The figure shows three views and two pictorial views of one solid part (mm, origin at its lowest corner). Answer the questions. A direction names the side the tool comes from. Coordinates: 2 decimals unless noted, no trailing zeros. Order: outer loops, then holes, each group sorted by start corner. A loop starts at its lowest first (then second) coordinate and runs counter-clockwise, first axis right, second up. Notation, with made-up numbers: (50.25, 75.5) - (74.25, 75.5) arc R16 ccw to (74.25, 100.5) - close; hole circle Ø3 at (83.25, 0.25). An arc over 180 degrees is marked (long way). Use one line per item in the form item = value.
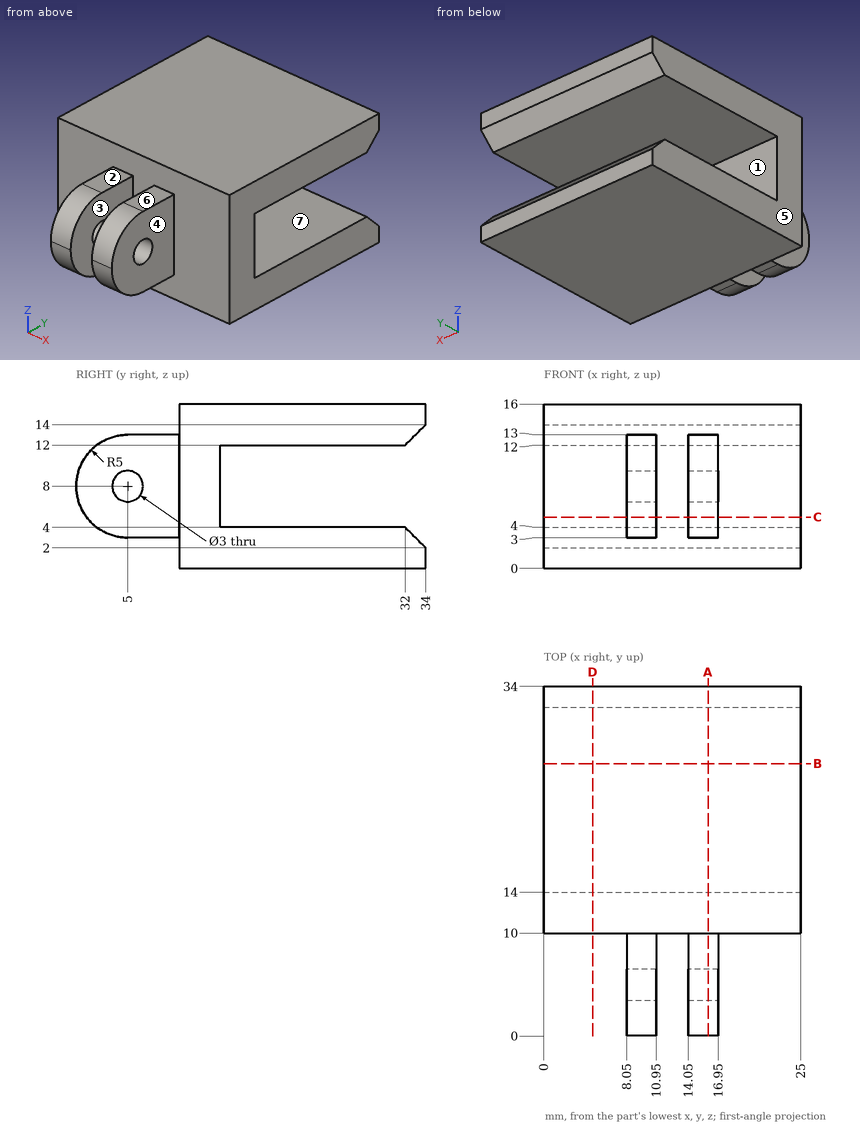
(1) Section B-B, the plane y = 26.5 is taken. Write down the section's boundary in (x, z), then the cut area to 3 significant figures.
Answer list:
outline = (0, 0) - (25, 0) - (25, 4) - (0, 4) - close; (0, 12) - (25, 12) - (25, 16) - (0, 16) - close
area = 200 mm2
(2) Given pin 1 Ø8 at (x, z) = (17, 7) entering from +Y; pin 2 Ø3 at (y, z) = (7.5, 6.5) entering from +X; pin 3 Ø0.9 at (x, y) = (15.5, 8.5) entering from -Z; pin 4 Ø9 at (x, y) = (11.5, 25) entering from -Z, each flat-ended and moving along its own axis, determine where each tip first touches the part or whether it passes through.
Answer list:
pin_1 = 33
pin_2 = 16.95
pin_3 = 3
pin_4 = 0
(3) Section A-A, the plane x = 16 is taken. Write down the section's boundary in (y, z).
Answer list:
outline = (5, 3) - (10, 3) - (10, 0) - (34, 0) - (34, 2) - (32, 4) - (14, 4) - (14, 12) - (32, 12) - (34, 14) - (34, 16) - (10, 16) - (10, 13) - (5, 13) arc R5 ccw to start; hole circle Ø3 at (5, 8)
(4) Which of the six approach directions +Z, -Z, +X, -X, +Y, -Y give full straight-line access (tool end or side, diameter ignored) to the marked faces 1, 2, 3 and 4?
Answer list:
face_1 = +X, -X, +Y
face_2 = +Z, +X, -X, -Y
face_3 = +Z, -Z, -Y
face_4 = +Z, -Z, +X, -Y
(5) The mould has two halves that part along Z. Classify the marked faces 5, 6 and 7: +Z half, -Z half, draft (parallel to the pull), parting line (faces both ways), or undercut.
Answer list:
face_5 = draft
face_6 = +Z half
face_7 = undercut
(6) Section D-D, the plane x = 4.75 is taken. Write down the section's boundary in (y, z), then the cut area to 3 significant figures.
Answer list:
outline = (10, 0) - (34, 0) - (34, 2) - (32, 4) - (14, 4) - (14, 12) - (32, 12) - (34, 14) - (34, 16) - (10, 16) - close
area = 220 mm2
(7) Straight lines are drawn through the part: L1, parallel to Z at x = 13.25, y = 31.5; L2, parallel to X at y = 9, z = 7.5; L3, parallel to Y at x = 23, z = 7.5. For each, find the intervals that lie inside material, in ascending order.
Answer list:
L1 = 0 to 4, 12 to 16
L2 = 8.05 to 10.95, 14.05 to 16.95
L3 = 10 to 14
(8) Section C-C, the plane z = 5 is taken. Write down the section's boundary in (x, y).
Answer list:
outline = (0, 10) - (8.05, 10) - (8.05, 1) - (10.95, 1) - (10.95, 10) - (14.05, 10) - (14.05, 1) - (16.95, 1) - (16.95, 10) - (25, 10) - (25, 14) - (0, 14) - close
